Could you check a few things on this model? Use its own coordinates, in mm. Face numbers are marked on the shaded views. A direction names the side the tool comes from. Give positions to 0.01 mm unless a question says otherwise; leave off trailing zeros. Order: outer loops, then holes, each group sorted by start corner. A loop starts at its lowest first (then second) coordinate and runs counter-clockwise, first axis right, second up.
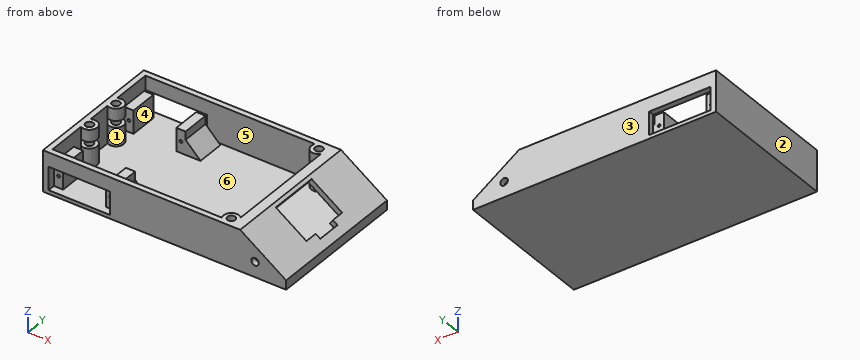
Autodesk Inventor part; units mm, degrees
ref_plane "Work Plane1" through (0, 66, 12.4) normal (0, 0, 1) x (1, 0, 0)
ref_plane "YZ Plane" through (0, 0, 0) normal (1, 0, 0) x (0, 1, 0)
ref_plane "XZ Plane" through (0, 0, 0) normal (0, 1, 0) x (-1, 0, 0)
sketch "Sketch1" plane through (0, 0, 0) normal (0, 0, 1) x (1, 0, 0)
  line L0 (0, 0) -> (100, 0)
  line L1 (100, 0) -> (100, 70)
  line L2 (100, 70) -> (0, 70)
  line L3 (0, 70) -> (0, 0)
  line L4 (-3, 73) -> (103, 73)
  line L5 (103, 73) -> (103, -3)
  line L6 (103, -3) -> (-3, -3)
  line L7 (-3, -3) -> (-3, 73)
  line L8 (100, 0) -> (103, 0)
  line L9 (100, 70) -> (103, 70)
  dimension "d0" = 100
  dimension "d1" = 70
  dimension "d2" = 3
extrude "Extrusion1" add sketch "Sketch1" against normal blind 2
extrude "Extrusion2" add sketch "Sketch1" along normal blind 20 contours L0 L8 L5 L6 L7 L4 L9 L2 L3 | L1 L9 L5 L8
sketch "Sketch2" plane through (0, 70, 0) normal (0, -1, 0) x (1, 0, 0)
  line L0 (0, 0) -> (0, 20)
  line L1 (100, 0) -> (0, 0)
  line L2 (0, 0) -> (33, 0)
  line L3 (33, 0) -> (33, 12.4)
  line L4 (33, 12.4) -> (0, 12.4)
  line L5 (0, 12.4) -> (0, 0)
  line L6 (100, 0) -> (0, 0)
  dimension "d7" = 33
  dimension "d8" = 12.4
extrude "Extrusion3" cut sketch "Sketch2" along normal through all both and the other way through all
sketch "Sketch3" plane through (0, 0, 0) normal (0, 0, 1) x (1, 0, 0)
  line L0 (33, 1) -> (28, 1)
  line L1 (28, 4) -> (28, 1)
  line L2 (0, 1) -> (5, 1)
  line L3 (5, 4) -> (5, 1)
  line L4 (5, 66) -> (5, 69)
  line L5 (0, 69) -> (5, 69)
  line L6 (33, 69) -> (28, 69)
  line L7 (28, 66) -> (28, 69)
  line L8 (33, 54) -> (28, 54)
  line L9 (28, 54) -> (28, 69)
  line L10 (28, 69) -> (33, 69)
  line L11 (33, 69) -> (33, 54)
  line L12 (5, 69) -> (0, 69)
  line L13 (0, 69) -> (0, 54)
  line L14 (0, 54) -> (5, 54)
  line L15 (5, 54) -> (5, 69)
  line L16 (0, 73) -> (0, -3)
  line L17 (0, 1) -> (5, 1)
  line L18 (5, 1) -> (5, 16)
  line L19 (5, 16) -> (0, 16)
  line L20 (0, 16) -> (0, 1)
  line L21 (33, 16) -> (28, 16)
  line L22 (28, 16) -> (28, 1)
  line L23 (28, 1) -> (33, 1)
  line L24 (33, 1) -> (33, 16)
  point P0 (0, 0)
  dimension "d11" = 15
  dimension "d12" = 15
  dimension "d13" = 15
  dimension "d14" = 15
ref_plane "Work Plane1" through (0, 66, 12.4) normal (0, 0, 1) x (1, 0, 0)
extrude "Extrusion4" add sketch "Sketch3" along normal up to surface (12.4 mm away)
sketch "Sketch4" plane through (28, 69, 0) normal (0, 1, 0) x (1, 0, 0)
  arc A0 (3.1614, -5.45) -> (3.1614, -6.95) centre (2.5, -6.2) ccw
  arc A1 (-26.1614, -6.95) -> (-26.1614, -5.45) centre (-25.5, -6.2) ccw
  point P0 (-28, 0)
hole "Hole1" at (30.5, 69, 6.2) at (2.5, 69, 6.2) direction (0, -1, 0) diameter 1.5 end through all
sketch "Sketch5" plane through (-3, 73, -2) normal (0, 1, 0) x (1, 0, 0)
  line L0 (106, -22) -> (0, -22)
  line L1 (106, -22) -> (106, 0)
  line L2 (0, 0) -> (106, 0)
  line L3 (106, -22) -> (106, 0)
  line L4 (106, -22) -> (130.7184, -5)
  line L5 (130.7184, -5) -> (130.7184, 0)
  line L6 (130.7184, 0) -> (106, 0)
  line L7 (104.4953, -19.3938) -> (127.7184, -3.4222)
  line L8 (127.7184, -3.4222) -> (127.7184, -3)
  line L9 (127.7184, -3) -> (106, -3)
  line L10 (106, -3) -> (106, 0)
  line L11 (106, -22) -> (100.7059, -22)
  line L12 (100.7059, -22) -> (104.4953, -19.3938)
  point P0 (3, -2)
  dimension "d32" = 30
  dimension "d33" = 5
  dimension "d42" = 3
extrude "Extrusion5" cut sketch "Sketch1" along normal through all contours L1 L9 L5 L8
extrude "Extrusion6" add sketch "Sketch5" against normal blind 76 contours L0 L12 L7 L1 | L1 L7 L8 L9 L6 L5 L4
extrude "Extrusion7" add sketch "Sketch5" against normal blind 3 contours L1 L7 L8 L9 L6 L5 L4 | L1 L9 L8 L7
sketch "Sketch6" plane through (-3, -3, -2) normal (0, -1, 0) x (1, 0, 0)
  line L0 (0, 0) -> (130.7184, 0)
  line L1 (130.7184, 5) -> (130.7184, 0)
  line L2 (106, 22) -> (130.7184, 5)
  line L3 (106, 22) -> (106, 0)
  point P0 (3, 2)
extrude "Extrusion8" add sketch "Sketch6" against normal blind 3
sketch "Sketch7" plane through (103, 0, 1) normal (-1, 0, 0) x (0, 0, 1)
  line L0 (-1, 0) -> (0, 0)
  line L1 (0, 70) -> (0, 0)
  line L2 (0, 70) -> (-1, 70)
  line L3 (-1, 70) -> (-1, 0)
  point P0 (-1, 0)
extrude "Extrusion9" cut sketch "Sketch7" against normal blind 21.75
sketch "Sketch8" plane through (127.7184, -3, 3) normal (0.5667, 0, 0.8239) x (0.8239, 0, -0.5667)
  line L0 (-28, 24.5) -> (-8, 24.5)
  line L1 (-8, 24.5) -> (-8, 51.5)
  line L2 (-8, 51.5) -> (-28, 51.5)
  line L3 (-28, 51.5) -> (-28, 24.5)
  line L4 (0, 76) -> (0, 0)
  line L5 (-30, 76) -> (0, 76)
  line L6 (-30, 0) -> (-30, 76)
  line L7 (0, 0) -> (-30, 0)
  line L8 (-28, 51.5) -> (-30, 76) construction
  line L9 (-30, 0) -> (-30, 76) construction
  line L10 (-28, 24.5) -> (-30, 0) construction
  line L11 (-8, 31.5) -> (-5, 31.5)
  line L12 (-5, 31.5) -> (-5, 44.5)
  line L13 (-5, 44.5) -> (-8, 44.5)
  line L14 (-8, 44.5) -> (-8, 31.5)
  line L15 (-8, 24.5) -> (-5, 31.5) construction
  line L16 (-5, 44.5) -> (-8, 51.5) construction
  point P0 (-103.5332, 3)
  dimension "d52" = 27
  dimension "d53" = 20
  dimension "d54" = 3
  dimension "d55" = 13
  dimension "d58" = 2
extrude "Extrusion10" cut sketch "Sketch8" against normal blind 3 contours L3 L2 L1 L0 | L1 L13 L12 L11
sketch "Sketch9" plane through (97.7059, 0, 20) normal (-0.5667, 0, -0.8239) x (-0.8239, 0, 0.5667)
  line L0 (-1.3621, 49.5) -> (-33.3621, 49.5)
  line L1 (-33.3621, 49.5) -> (-33.3621, 20.5)
  line L2 (-33.3621, 20.5) -> (-1.3621, 20.5)
  line L3 (-1.3621, 20.5) -> (-1.3621, 49.5)
  line L4 (-6.3621, 48.5) -> (-6.3621, 21.5)
  line L5 (-29.3621, 28.5) -> (-29.3621, 41.5)
  point P0 (69.1711, 0)
  dimension "d59" = 5
  dimension "d60" = 4
  dimension "d61" = 1
  dimension "d62" = 1
sketch "Sketch10" plane through (0, 0, 20) normal (0, 0, 1) x (1, 0, 0)
  point P0 (0, 0)
sketch "Sketch12" plane through (-3, -3, -2) normal (0, -1, 0) x (1, 0, 0)
  circle A0 centre (14, 8.2) radius 1.0065 construction
  line L0 (14, 8.2) -> (114, 8.2)
  circle A1 centre (114, 8.2) radius 2
  point P0 (3, 2)
  dimension "d67" = 100
  dimension "d68" = 4
extrude "Extrusion12" cut sketch "Sketch12" against normal through all
sketch "Sketch13" plane through (0, 0, 0) normal (0, 0, 1) x (1, 0, 0)
  circle A0 centre (2, 25) radius 2.125
  circle A1 centre (2, 45) radius 2.125
  line L0 (97.7059, 0) -> (0, 0)
  line L1 (0, 70) -> (97.7059, 70)
  line L2 (0, 0) -> (0, 70)
  circle A2 centre (2, 25) radius 4.125
  circle A3 centre (2, 45) radius 4.125
  dimension "d71" = 25
  dimension "d72" = 25
  dimension "d73" = 2
  dimension "d74" = 4.25
  dimension "d75" = 4.25
  dimension "d76" = 2
  dimension "d77" = 2
  dimension "d78" = 2
extrude "Extrusion13" add sketch "Sketch13" along normal up to surface (20 mm away)
extrude "Extrusion14" cut sketch "Sketch13" along normal up to surface (20 mm away) contours A0 L2 | L2 A0 | L2 A1 | A1 L2
sketch "Sketch14" plane through (0, 0, 0) normal (0, 0, 1) x (1, 0, 0)
  circle A0 centre (94.7059, 2) radius 2.125
  circle A1 centre (94.7059, 68) radius 2.125
  circle A2 centre (94.7059, 2) radius 4.125
  circle A3 centre (94.7059, 68) radius 4.125
  line L0 (97.7059, 0) -> (0, 0)
  line L1 (33, 70) -> (124.75, 70)
  line L2 (97.7059, 70) -> (97.7059, 0)
  dimension "d83" = 4.25
  dimension "d84" = 4.25
  dimension "d85" = 2
  dimension "d86" = 2
  dimension "d87" = 2
  dimension "d88" = 2
  dimension "d89" = 3
  dimension "d90" = 3
extrude "Extrusion15" add sketch "Sketch14" along normal up to surface (20 mm away)
extrude "Extrusion16" cut sketch "Sketch14" along normal up to surface (20 mm away) contours A0 L0 | L0 A0 | L1 A1 | A1 L1
ref_plane "Work Plane2" through (0, 0, 10) normal (0, 0, 1) x (1, 0, 0)
sketch "Sketch15" plane through (0, 0, 10) normal (0, 0, 1) x (1, 0, 0)
  arc A0 (91.0982, 70) -> (98.3136, 70) centre (94.7059, 68) ccw
  circle A1 centre (94.7059, 2) radius 4.125
  circle A2 centre (94.7059, 68) radius 4.125
  circle A3 centre (2, 25) radius 4.125
  circle A4 centre (2, 45) radius 4.125
  circle A5 centre (2, 25) radius 2.125 construction
  circle A6 centre (2, 45) radius 2.125 construction
  circle A7 centre (94.7059, 2) radius 2.125 construction
  circle A8 centre (94.7059, 68) radius 2.125 construction
  arc A9 (98.3136, 0) -> (91.0982, 0) centre (94.7059, 2) ccw construction
  arc A10 (0, 21.3923) -> (0, 28.6077) centre (2, 25) ccw construction
  arc A11 (0, 41.3923) -> (0, 48.6077) centre (2, 45) ccw construction
  point P0 (0, 0)
extrude "Extrusion17" cut sketch "Sketch15" along normal blind 3.5
chamfer "Chamfer1" distance 8 angle 45 2 edges at (33, 61.5, 0) (33, 8.5, 0)
equation "\"d12\" = d11"
equation "\"d13\" = d11"
equation "\"d14\" = d11"
equation "\"d62\" = d61"
equation "\"d72\" = d71"
equation "\"d75\" = d74"
equation "\"d76\" = d73"
equation "\"d88\" = d87"
equation "\"d90\" = d89"
properties part number "base" material "Ogólne"
Item 1: Imagine slicing it at B-B on y = 59. Give the number of separate pieces and of enclosed holes in the cut face, then the cut area to 3 significant figures.
Findings:
separate pieces: 1
enclosed holes: 2
area: 575 mm2
Item 2: Please list where these lines run through material, in increasing order: line 1 along Z through (x, y) = (2.5, 4.5); line 2 along Y through (x, z) = (114, 5.5); line 3 along X through (y, z) = (25, 5.75) (3 decimals).
Findings:
line 1: z = -2 to 5.45, 6.95 to 12.4
line 2: y = -3 to 0, 70 to 73
line 3: x = -3 to -0.125, 4.125 to 6.125, 119.9 to 123.72
Item 3: Imagine slicing it at A-A on x = 24. List the corners of the cut face in (y, z) for me.
Findings:
outline: (-3, -2) - (73, -2) - (73, 0) - (-3, 0) - close; (-3, 12.4) - (0, 12.4) - (0, 20) - (-3, 20) - close; (70, 12.4) - (73, 12.4) - (73, 20) - (70, 20) - close
Item 4: For pin 1 (2.5 mm diameter, centred on x = 31.5, y = 7.5, fed in from +Z); pin 2 (1.3 mm diameter, centred on y = 62.5, z = 10, fed in from +X); pin 3 (3.5 mm diameter, centred on y = 5.5, z = 8.5, fed in from +X), each with a flat end and sliding along its axis, tell me the tip position at first contact or that it passes through.
Findings:
pin 1: stops at z = 12.4
pin 2: stops at x = 118.49
pin 3: stops at x = 122.27
Item 5: For the marked faces 4, 5 and 6, which set-ups out of +Z, -Z, +X, -X, +Y, -Y let a thin tool reach every point of the face, with its end or its side?
Findings:
face 4: +Z, +Y
face 5: +Z
face 6: none
Item 6: We'd pull the mould along Y, two halves only. Please class the marked faces 1, 2 and 3: +Y half, -Y half, draft (parallel to the pull), parting line (faces both ways), or undercut.
Findings:
face 1: undercut
face 2: draft
face 3: +Y half
